Part model, mm, in its own coordinate system. A direction names the side the tool comes from. Coordinates: 2 decimals unless noted, no trailing zeros. Loops run counter-clockwise (first coordinate to the right, second up) from the corner with the lowest first, then second, coordinate; pieces in that order, holes last. Notation, with made-up numbers: M 43,-8 L 73,-8 A15 cw 73,13 Z; hole C 2.25,31.25 d9. An arc over 180 degrees is marked long. Answer as a JSON object with one key per item and string values. Group by question number.
1. Saw through at D-D on z = 9. Write the cut outline in (x, y), then the cut area to 3 significant figures.
2. Saw through at A-A on x = 0. Write the cut outline in (y, z) (3 decimals), then the cut area to 3 significant figures.
3. 3-axis set-ups, long thin cutter, end or side, ignore diameter. For faces 4 (the face through (-0.794, 15.357, -6.044)), 5 (the face through (3, 0, 3)): which of +Z, -Z, +X, -X, +Y, -Y reach the whole face in a straight line?
4. Drill centre lines: L1, parallel to Z at x = 0, y = 11.25; L2, parallel to Y at x = -8.75, z = -4; L3, parallel to Z at x = -1, y = 3.25. Where is each one in solid material? Low to high.
5. Drop flat-ended pins along their axis: pin 1 Ø6 at (x, y) = (3, 11.5) entering from -Z; pin 2 Ø3 at (x, z) = (9, -3.5) entering from -Y; pin 3 Ø8 at (x, z) = (-9.5, 9) entering from +Y; pin 4 Ø6 at (y, z) = (15.5, 7) entering from +X. Give the stop position or say it passes through.
6. Mould opens along X. For faces 1 (the face through (-2.75, 0.63, 12.4)), 2 (the face through (5.5, 1.27, -3)), 3 (the face through (0.708, 14.714, 3.186)) say: released by +X, released by -X, zero draft, split by the parting line, or undercut.
7. Saw through at B-B on z = 0. Write the cut outline in (x, y) (3 decimals).
8. Saw through at C-C on y = 6. Write the cut outline in (x, z), then the cut area to 3 significant figures.
from build123d import *

# Parameters (mm, degrees)
SKETCH1_R                = 12.7
BOSS_EXTRUDE1_DEPTH      = 1.27
SKETCH2_R                = 6.096
BOSS_EXTRUDE2_DEPTH      = 28.575
F_5_16_18_TAPPED_HOLE1_D = 6.5278


with BuildPart() as part:
    # Sketch1 → Boss-Extrude1 (new body)
    with BuildSketch(Plane(origin=(0, 0, 0), x_dir=(1, 0, 0), z_dir=(0, 1, 0))):
        Circle(SKETCH1_R)
    extrude(amount=BOSS_EXTRUDE1_DEPTH)

    # Sketch2 → Boss-Extrude2 (add)
    with BuildSketch(Plane(origin=(0, 1.27, 0), x_dir=(1, 0, 0), z_dir=(0, 1, 0))):
        Circle(SKETCH2_R)
    extrude(amount=BOSS_EXTRUDE2_DEPTH)

    # 5/16-18 Tapped Hole1 (through all)
    with Locations(Plane(origin=(0, 29.845, 0), x_dir=(1, 0, 0), z_dir=(0, 1, 0))):
        with Locations((0, 0)):
            Hole(F_5_16_18_TAPPED_HOLE1_D / 2)


solid = part.part
Outcome:
{
 "1": {"outline": "M -8.96,0 L 8.96,0 L 8.96,1.27 L -8.96,1.27 Z", "area": "22.8 mm²"},
 "2": {"outline": "M 0,-12.7 L 1.27,-12.7 L 1.27,-6.096 L 29.845,-6.096 L 29.845,-3.264 L 0,-3.264 Z; M 0,3.264 L 29.845,3.264 L 29.845,6.096 L 1.27,6.096 L 1.27,12.7 L 0,12.7 Z", "area": "186 mm²"},
 "3": {"face 4": "+Y", "face 5": "+Z, -Z, +X, -X, -Y"},
 "4": {"L1": "z = -6.1 to -3.26, 3.26 to 6.1", "L2": "y = 0 to 1.27", "L3": "z = -6.01 to -3.11, 3.11 to 6.01"},
 "5": {"pin 1": "stops at z = -6.1", "pin 2": "stops at y = 0", "pin 3": "stops at y = 1.27", "pin 4": "stops at x = 4.6"},
 "6": {"face 1": "split by the parting line", "face 2": "zero draft", "face 3": "undercut"},
 "7": {"outline": "M -12.7,0 L -3.264,0 L -3.264,29.845 L -6.096,29.845 L -6.096,1.27 L -12.7,1.27 Z; M 3.264,0 L 12.7,0 L 12.7,1.27 L 6.096,1.27 L 6.096,29.845 L 3.264,29.845 Z"},
 "8": {"outline": "C 0,0 d12.19; hole C 0,0 d6.53", "area": "83.3 mm²"}
}
